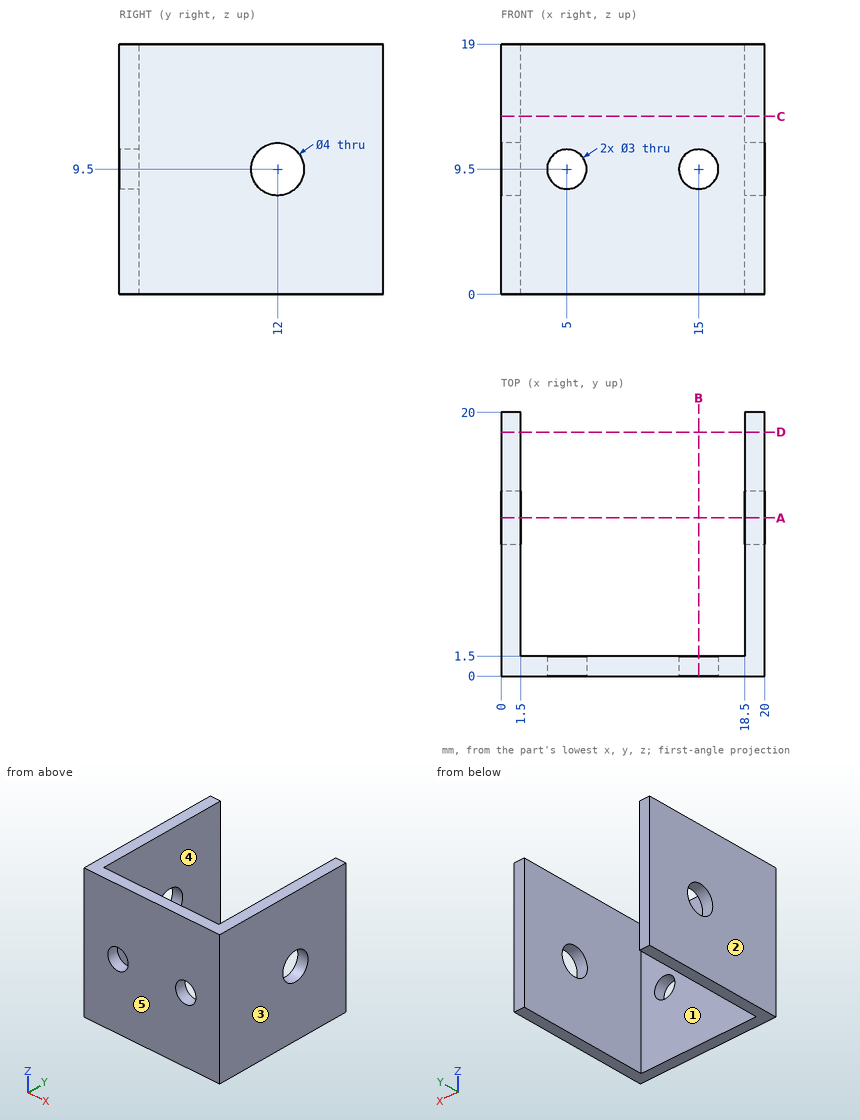
Verification items for this drawing (mm, ordinates from the low corner). A direction names the side the tool comes from. Give positions to 0.01 mm unless a question says otherwise; leave off trailing zeros. Write each loop counter-clockwise with the first axis right and the second up, starting at its lowest first coordinate (ties: lowest second). Pieces come first, ordered by that corner, then holes. Notation, with made-up numbers: M 70.5,48.5 L 106.5,48.5 A38 cw 106.5,86.5 Z; hole C 68,-33.5 d3. An arc over 180 degrees is marked long. Use one line per item in the form item = value.
(1) Section check A-A on y = 12. Record the boundary of the cut face in (x, z).
Answer block:
outline = M 0,0 L 1.5,0 L 1.5,7.5 L 0,7.5 Z; M 0,11.5 L 1.5,11.5 L 1.5,19 L 0,19 Z; M 18.5,0 L 20,0 L 20,7.5 L 18.5,7.5 Z; M 18.5,11.5 L 20,11.5 L 20,19 L 18.5,19 Z
(2) Section check C-C on z = 13.5. Record the boundary of the cut face in (x, y).
Answer block:
outline = M 0,0 L 20,0 L 20,20 L 18.5,20 L 18.5,1.5 L 1.5,1.5 L 1.5,20 L 0,20 Z
(3) Tool access check on the marked faces 1 and 2. Record the directions out of +Z, -Z, +X, -X, +Y, -Y that give a thin tool (end or side, any length) a straight path to the whole face; none if there is none.
Answer block:
face_1 = +Z, -Z, +Y
face_2 = +Z, -Z, -X, +Y, -Y
(4) Material ranges on line 1 along X through (y, z) = (10, 13.25); line 2 along Z through (x, y) = (19.45, 12); line 3 along Y through (x, z) = (10, 4.5), recorded low to high.
Answer block:
line_1 = 0 to 1.5, 18.5 to 20
line_2 = 0 to 7.5, 11.5 to 19
line_3 = 0 to 1.5
(5) Section check B-B on x = 15. Record the boundary of the cut face in (y, z).
Answer block:
outline = M 0,0 L 1.5,0 L 1.5,8 L 0,8 Z; M 0,11 L 1.5,11 L 1.5,19 L 0,19 Z
(6) Section check D-D on y = 18.5. Record the boundary of the cut face in (x, z).
Answer block:
outline = M 0,0 L 1.5,0 L 1.5,19 L 0,19 Z; M 18.5,0 L 20,0 L 20,19 L 18.5,19 Z
(7) Depth check by flat-ended pin: P1, Ø5, axis at x = 7.5, z = 12, coming from the +Y side; P2, Ø6, axis at x = 7, y = 14, coming from the +Z side; P3, Ø6, axis at y = 15, z = 15, coming from the -X side. Enter the tip coordinate at first touch or a pass-through.
Answer block:
P1 = 1.5
P2 = through
P3 = 0
(8) Draft check along X on the marked faces 3, 4 and 5. Enter one of: pulls with the +X half, pulls with the -X half, needs draft (parallel to the pull), parting line crosses it, or undercut.
Answer block:
face_3 = pulls with the +X half
face_4 = undercut
face_5 = needs draft
